Model file for the job. Use its own axes, mm. A direction names the side the tool comes from. Give positions to 0.01 mm unless a question says otherwise; leave off trailing zeros. Loops run counter-clockwise (first coordinate to the right, second up) from the corner with the lowest first, then second, coordinate; pieces in that order, holes last. Notation, with made-up numbers: M 39,-17.75 L 83,-17.75 A29 cw 83,5.25 Z; hole C -22.75,43 d2. An arc over 180 degrees is marked long. Answer in a Markdown table with one row per item.
```python
from build123d import *

# Parameters (mm, degrees)
SKETCH1_W            = 30
SKETCH1_H            = 30
BOSS_EXTRUDE1_DEPTH  = 6
BOSS_EXTRUDE4_DEPTH  = 20
SKETCH4_W            = 2
SKETCH4_H            = 2
BOSS_EXTRUDE6_DEPTH  = 20
SKETCH5_W            = 24
SKETCH5_H            = 6
BOSS_EXTRUDE7_DEPTH  = 20
SHELL2_START         = 7
SHELL2_DEPTH         = 23
SHELL2_START_2       = 1
SHELL2_2_DEPTH       = 4
SHELL2_START_3       = 5
SHELL2_3_OUTLINE_W   = 29
SHELL2_3_OUTLINE_H   = 4
SHELL2_3_DEPTH       = 2
SKETCH7_W            = 23
SKETCH7_H            = 1
BOSS_EXTRUDE8_DEPTH  = 5
SKETCH9_W            = 1.075143629
SKETCH9_H            = 23
BOSS_EXTRUDE9_DEPTH  = 5
SKETCH10_W           = 4
SKETCH10_H           = 23
CUT_EXTRUDE1_DEPTH   = 10
SKETCH11_W           = 23
SKETCH11_H           = 4
CUT_EXTRUDE2_DEPTH   = 10
BOSS_EXTRUDE10_DEPTH = 20
SKETCH13_W           = 20
SKETCH13_H           = 4
CUT_EXTRUDE3_DEPTH   = 5
SKETCH14_W           = 30
SKETCH14_H           = 26
BOSS_EXTRUDE11_DEPTH = 0.5
SKETCH15_W           = 26
SKETCH15_H           = 30.5
BOSS_EXTRUDE12_DEPTH = 0.5
SKETCH16_W           = 20
SKETCH16_H           = 24
BOSS_EXTRUDE13_DEPTH = 0.5
SKETCH19_W           = 30.5
SKETCH19_H           = 30.5
BOSS_EXTRUDE14_DEPTH = 0.5
SKETCH20_W           = 23.5
SKETCH20_H           = 24
BOSS_EXTRUDE15_DEPTH = 0.5
SKETCH21_W           = 23.5
SKETCH21_H           = 19.5
BOSS_EXTRUDE16_DEPTH = 0.5
SKETCH25_W           = 28
SKETCH25_H           = 4
BOSS_EXTRUDE17_DEPTH = 0.5


# Read off the part's stored shape, not the designer's step: Shell2
with BuildPart() as part:
    # Sketch1 → Boss-Extrude1 (new body)
    with BuildSketch(Plane.XY):
        with Locations((15, 15)):
            Rectangle(SKETCH1_W, SKETCH1_H)
    extrude(amount=BOSS_EXTRUDE1_DEPTH)

    # Sketch2 → Boss-Extrude4 (add)
    with BuildSketch(Plane.XY.offset(6)):
        Polygon((5, 6), (6, 6), (6, 30), (0, 30), (0, 6), align=None)
    extrude(amount=BOSS_EXTRUDE4_DEPTH)

    # Sketch4 → Boss-Extrude6 (add)
    with BuildSketch(Plane.XY.offset(6)):
        with Locations((5, 5)):
            Rectangle(SKETCH4_W, SKETCH4_H)
    extrude(amount=BOSS_EXTRUDE6_DEPTH)

    # Sketch5 → Boss-Extrude7 (add)
    with BuildSketch(Plane.XY.offset(6)):
        with Locations((18, 3)):
            Rectangle(SKETCH5_W, SKETCH5_H)
    extrude(amount=BOSS_EXTRUDE7_DEPTH)

    # Shell2 outline → Shell2 (cut)
    with BuildSketch(Plane(origin=(0, 0, 0), x_dir=(1, 0, 0), z_dir=(0, 1, 0)).offset(SHELL2_START)):
        Polygon((5, -5), (30, -5), (30, -1), (1, -1), (1, -25), (5, -25), align=None)
    extrude(amount=SHELL2_DEPTH, mode=Mode.SUBTRACT)

    # Shell2 2 outline → Shell2 2 (cut)
    with BuildSketch(Plane(origin=(0, 0, 0), x_dir=(1, 0, 0), z_dir=(0, 1, 0)).offset(SHELL2_START_2)):
        Polygon((7, -5), (7, -25), (30, -25), (30, -1), (1, -1), (1, -5), align=None)
    extrude(amount=SHELL2_2_DEPTH, mode=Mode.SUBTRACT)

    # Shell2 3 outline → Shell2 3 (cut)
    with BuildSketch(Plane(origin=(0, 0, 0), x_dir=(1, 0, 0), z_dir=(0, 1, 0)).offset(SHELL2_START_3)):
        with Locations((15.5, -3)):
            Rectangle(SHELL2_3_OUTLINE_W, SHELL2_3_OUTLINE_H)
    extrude(amount=SHELL2_3_DEPTH, mode=Mode.SUBTRACT)

    # Sketch7 → Boss-Extrude8 (add)
    with BuildSketch(Plane.XZ.offset(-5)):
        with Locations((18.5, 5.5)):
            Rectangle(SKETCH7_W, SKETCH7_H)
    extrude(amount=BOSS_EXTRUDE8_DEPTH)

    # Sketch9 → Boss-Extrude9 (add)
    with BuildSketch(Plane.ZY.offset(-5)):
        with Locations((5.537571814, 18.5)):
            Rectangle(SKETCH9_W, SKETCH9_H)
    extrude(amount=BOSS_EXTRUDE9_DEPTH)

    # Sketch10 → Cut-Extrude1 (cut)
    with BuildSketch(Plane.XY.offset(26)):
        with Locations((3, 18.5)):
            Rectangle(SKETCH10_W, SKETCH10_H)
    extrude(amount=-CUT_EXTRUDE1_DEPTH, mode=Mode.SUBTRACT)

    # Sketch11 → Cut-Extrude2 (cut)
    with BuildSketch(Plane.XY.offset(26)):
        with Locations((18.5, 3)):
            Rectangle(SKETCH11_W, SKETCH11_H)
    extrude(amount=-CUT_EXTRUDE2_DEPTH, mode=Mode.SUBTRACT)

    # Sketch12 → Boss-Extrude10 (add)
    with BuildSketch(Plane.XY.offset(6)):
        Polygon((6, 0), (6, 4), (4, 4), (4, 6), (0, 6), (0, 0), align=None)
    extrude(amount=BOSS_EXTRUDE10_DEPTH)

    # Sketch13 → Cut-Extrude3 (cut)
    with BuildSketch(Plane(origin=(7, 0, 0), x_dir=(0, 0, -1), z_dir=(1, 0, 0))):
        with Locations((-16, 3)):
            Rectangle(SKETCH13_W, SKETCH13_H)
    extrude(amount=-CUT_EXTRUDE3_DEPTH, mode=Mode.SUBTRACT)

    # Sketch14 → Boss-Extrude11 (add)
    with BuildSketch(Plane.XZ):
        with Locations((15, 13)):
            Rectangle(SKETCH14_W, SKETCH14_H)
    extrude(amount=BOSS_EXTRUDE11_DEPTH)

    # Sketch15 → Boss-Extrude12 (add)
    with BuildSketch(Plane.ZY):
        with Locations((13, 14.75)):
            Rectangle(SKETCH15_W, SKETCH15_H)
    extrude(amount=BOSS_EXTRUDE12_DEPTH)

    # Sketch16 → Boss-Extrude13 (add)
    with BuildSketch(Plane(origin=(6, 0, 0), x_dir=(0, 0, -1), z_dir=(1, 0, 0))):
        with Locations((-16, 18)):
            Rectangle(SKETCH16_W, SKETCH16_H)
    extrude(amount=BOSS_EXTRUDE13_DEPTH)

    # Sketch19 → Boss-Extrude14 (add)
    with BuildSketch(Plane(origin=(0, 0, 0), x_dir=(-1, 0, 0), z_dir=(0, 0, -1))):
        with Locations((-14.75, 14.75)):
            Rectangle(SKETCH19_W, SKETCH19_H)
    extrude(amount=BOSS_EXTRUDE14_DEPTH)

    # Sketch20 → Boss-Extrude15 (add)
    with BuildSketch(Plane.XY.offset(6)):
        with Locations((18.25, 18)):
            Rectangle(SKETCH20_W, SKETCH20_H)
    extrude(amount=BOSS_EXTRUDE15_DEPTH)

    # Sketch21 → Boss-Extrude16 (add)
    with BuildSketch(Plane(origin=(0, 6, 0), x_dir=(1, 0, 0), z_dir=(0, 1, 0))):
        with Locations((18.25, -16.25)):
            Rectangle(SKETCH21_W, SKETCH21_H)
    extrude(amount=BOSS_EXTRUDE16_DEPTH)

    # Sketch25 → Boss-Extrude17 (add)
    with BuildSketch(Plane.XY.offset(6)):
        with Locations((16, 3)):
            Rectangle(SKETCH25_W, SKETCH25_H)
    extrude(amount=BOSS_EXTRUDE17_DEPTH)


solid = part.part
```
(1) Mould opens along Y. For faces 1 (the flat face through (16, 3, 6.5)), 2 (the flat face through (6.5, 18, 16)), 3 (the flat face through (15, 1, 3)) say: pulls with the +Y half, pulls with the -Y half, needs draft (parallel to the pull), parting line crosses it, or undercut.
Established:
| item | result |
|---|---|
| face 1 | undercut |
| face 2 | needs draft |
| face 3 | pulls with the +Y half |
(2) Wall check: L1, parallel to Z at x = 16, y = 14; L2, parallel to Y at x = 5.5, z = 16.25. Give the ranges that are in metal, low to high.
Established:
| item | result |
|---|---|
| L1 | z = -0.5 to 1, 5 to 6.5 |
| L2 | y = -0.5 to 1, 5 to 30 |
(3) Flat gauge pins, fed straight in: P1, Ø1.2, axis at x = 2.5, y = 13.5, coming from the +Z side; P2, Ø1.5, axis at x = 2.5, z = 12.5, coming from the +Y side; P3, Ø1.2, axis at x = 14, y = 3.5, coming from the +Z side. Where does each tip first touch, or does it go through?
Established:
| item | result |
|---|---|
| P1 | stops at z = 6.08 |
| P2 | stops at y = 7 |
| P3 | stops at z = 6.5 |
(4) Which spindle directions (+Z, -Z, +X, -X, +Y, -Y) get a long thin tool onto all of the face, cutting with end or side? Do faces 4 (the flat face through (18, 18, 6.5)), 5 (the flat face through (3, 18, 6.075)), 6 (the flat face through (16, 1, 16)). Say none if no direction does.
Established:
| item | result |
|---|---|
| face 4 | +Z, +X, +Y |
| face 5 | +Z, +Y |
| face 6 | +Z, +X |
(5) Saw through at A-A, the plane y = 24. Give the cut face in (x, z).
Established:
| item | result |
|---|---|
| outline | M -0.5,-0.5 L 30,-0.5 L 30,1 L 1,1 L 1,5 L 30,5 L 30,6.5 L 6.5,6.5 L 6.5,26 L 5,26 L 5,6.08 L 1,6.08 L 1,26 L -0.5,26 Z |
(6) Saw through at C-C, the plane z = 3.75. Give the cut face in (x, y), and give its area (4 significant figures).
Established:
| item | result |
|---|---|
| outline | M -0.5,-0.5 L 30,-0.5 L 30,1 L 1,1 L 1,30 L -0.5,30 Z |
| area | 89.25 mm2 |
(7) Saw through at B-B, the plane x = 11.5. Give the cut face in (y, z).
Established:
| item | result |
|---|---|
| outline | M -0.5,-0.5 L 30,-0.5 L 30,1 L 1,1 L 1,5 L 30,5 L 30,6.5 L 6.5,6.5 L 6.5,26 L 5,26 L 5,6.5 L 1,6.5 L 1,26 L -0.5,26 Z |
